Work out the finished part from the listing and answer in its coordinate system (mm). Face numbers are marked on the shaded views. A direction names the side the tool comes from. Coordinates: 2 decimals unless noted, no trailing zeros. Order: outer loops, then holes, each group sorted by start corner. A loop starts at its lowest first (then second) coordinate and runs counter-clockwise, first axis right, second up. Notation, with made-up numbers: (87, -13) - (101, -13) arc R32 cw to (101, 20) - close; hole circle Ø5 at (-29, -8). An arc over 180 degrees is marked (long way). Use CSV: the item, a comma, the result in double quotes. Start each with the question number.
Autodesk Inventor part; units mm, degrees
ref_plane "YZ Plane" through (0, 0, 0) normal (1, 0, 0) x (0, 1, 0)
ref_plane "XZ Plane" through (0, 0, 0) normal (0, 1, 0) x (-1, 0, 0)
ref_plane "XY Plane" through (0, 0, 0) normal (0, 0, 1) x (1, 0, 0)
sketch "Sketch1" plane through (0, 0, 0) normal (1, 0, 0) x (0, 1, 0)
  circle A0 centre (0, 0) radius 30.1625
  circle A1 centre (0, 0) radius 10.16 construction
  line L0 (7.3323, 0) -> (3.6662, -6.35)
  line L1 (3.6662, -6.35) -> (-3.6662, -6.35)
  line L2 (-3.6662, -6.35) -> (-7.3323, 0)
  line L3 (-7.3323, 0) -> (-3.6662, 6.35)
  line L4 (-3.6662, 6.35) -> (3.6662, 6.35)
  line L5 (3.6662, 6.35) -> (7.3323, 0)
  dimension "d0" = 60.325
  dimension "d1" = 20.32
  dimension "d2" = 12.7
extrude "Extrusion1" add sketch "Sketch1" along normal blind 10.16
sketch "Sketch2" plane through (10.16, 0, 0) normal (1, 0, 0) x (0, 0, -1)
  circle A0 centre (0, 0) radius 22.5425
  circle A1 centre (0, 0) radius 10.16
  dimension "d5" = 45.085
  dimension "d6" = 20.32
extrude "Extrusion2" cut sketch "Sketch2" against normal blind 3.175
sketch "Sketch3" plane through (0, 0, 0) normal (-1, 0, 0) x (0, 0, 1)
  circle A0 centre (0, 0) radius 10.16
  circle A1 centre (0, 0) radius 22.5425
  dimension "d9" = 20.32
  dimension "d10" = 45.085
extrude "Extrusion3" cut sketch "Sketch3" against normal blind 3.175
properties part number "banebots 400 - 2 3-8 replacement"
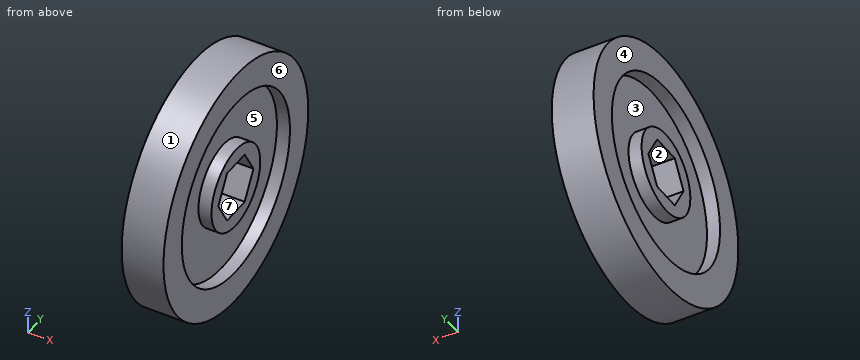
1) For a pull along Z with two mould halves and no side action, classify the marked faces 1, 2, 3 and 4 as +Z half, -Z half, draft (parallel to the pull), parting line (faces both ways), or undercut.
2) The part is cut by section D-D on z = 1.5. Determine the outline of the cut face in (x, y) (3 decimals), plus the area to 3 significant figures.
3) Straight lines are drawn through the part: line 1 (Y direction, x = 8.75, z = -4.5); line 2 (X direction, y = 4, z = 22) (3 decimals); line 3 (Y direction, x = 3, z = -8). For each, find the intervals that lie inside material, in ascending order. Write a range as [from, to].
4) For the marked faces 5, 6 and 7, determine the directions among +Z, -Z, +X, -X, +Y, -Y from which every point of the face is accessible in a straight line to the end or side of a thin tool.
5) Flat-ended cylindrical pins translate along their axes: P1, Ø2, axis at x = 3, y = 1.5, coming from the -Z side; P2, Ø3, axis at y = -3.5, z = -12, coming from the +X side (3 decimals); P3, Ø6, axis at x = 3, z = -12, coming from the +Y side; P4, Ø1, axis at y = 23.5, z = -13, coming from the -X side. Find the tip coordinate at first contact, or state that the pin passes through.
6) The part is cut by section A-A on x = 9. State how many separate pieces and enclosed holes the cut face has, plus the area to 3 significant figures.
Answer key:
1,face 1,"parting line"
1,face 2,"undercut"
1,face 3,"undercut"
1,face 4,"draft"
2,outline,"(0, -30.125) - (10.16, -30.125) - (10.16, -22.493) - (6.985, -22.493) - (6.985, -10.049) - (10.16, -10.049) - (10.16, -6.466) - (0, -6.466) - (0, -10.049) - (3.175, -10.049) - (3.175, -22.493) - (0, -22.493) - close; (0, 6.466) - (10.16, 6.466) - (10.16, 10.049) - (6.985, 10.049) - (6.985, 22.493) - (10.16, 22.493) - (10.16, 30.125) - (0, 30.125) - (0, 22.493) - (3.175, 22.493) - (3.175, 10.049) - (0, 10.049) - close"
2,area,"323 mm^2"
3,line 1,"[-29.82, -22.09], [-9.11, -4.73], [4.73, 9.11], [22.09, 29.82]"
3,line 2,"[3.175, 6.985]"
3,line 3,"[-29.08, -21.08], [-6.26, 6.26], [21.08, 29.08]"
4,face 5,"+X"
4,face 6,"+Z, -Z, +X, +Y, -Y"
4,face 7,"+X, -X"
5,P1,"z = -30.16"
5,P2,"x = 6.985"
5,P3,"y = 28.79"
5,P4,"x = 0"
6,separate pieces,"2"
6,enclosed holes,"2"
6,area,"1,450 mm^2"
